Here's the drawing with two shaded views (mm, measured from the low corner). I have some questions. A direction names the side the tool comes from. Coordinates: 2 decimals unless noted, no trailing zeros. Loops run counter-clockwise (first coordinate to the right, second up) from the corner with the lowest first, then second, coordinate; pieces in that order, holes last. Notation, with made-up numbers: (-32, 7.25) -> (7, 7.25) arc R20 ccw to (7, 41.25) -> close; hole circle Ø10 at (5, 87). An arc over 180 degrees is marked (long way). Answer as a JSON object with one key per item and string values. Group by question number.
Q1. I want a section at C-C on y = 22. Write out the boundary of the cut face in (x, z).
Q2. I want a section at A-A on x = 26. Write out the boundary of the cut face in (y, z) (1 decimal), then the cut area to 3 significant figures.
Q3. On a 3-axis mill with a long thin cutter (end or side, diameter ignored), from which of +Z, -Z, +X, -X, +Y, -Y can I reach the whole of each face in a straight line? I mean the marked faces 1 and 2. Say none if no direction works.
Q4. I want a section at B-B on z = 11.5. Write out the boundary of the cut face in (x, y), then the cut area to 3 significant figures.
Q5. I want a section at D-D on x = 67. Write out the boundary of the cut face in (y, z) (1 decimal), then the cut area to 3 significant figures.
Q6. I need wall thicknesses on line 1 (Y direction, x = 29.5, z = 40); line 2 (Z direction, x = 21, y = 10); line 3 (X direction, y = 16, z = 22) (1 decimal). Which ranges of each line are inside material? Lowest first, please.
Q7. I'm going to push flat-ended pins straight in: pin 1 (6 mm diameter, centred on x = 49, y = 42.5, fed in from -Z); pin 2 (1 mm diameter, centred on x = 38.5, z = 49, fed in from -Y). Where does each tip first touch, or does it pass through?
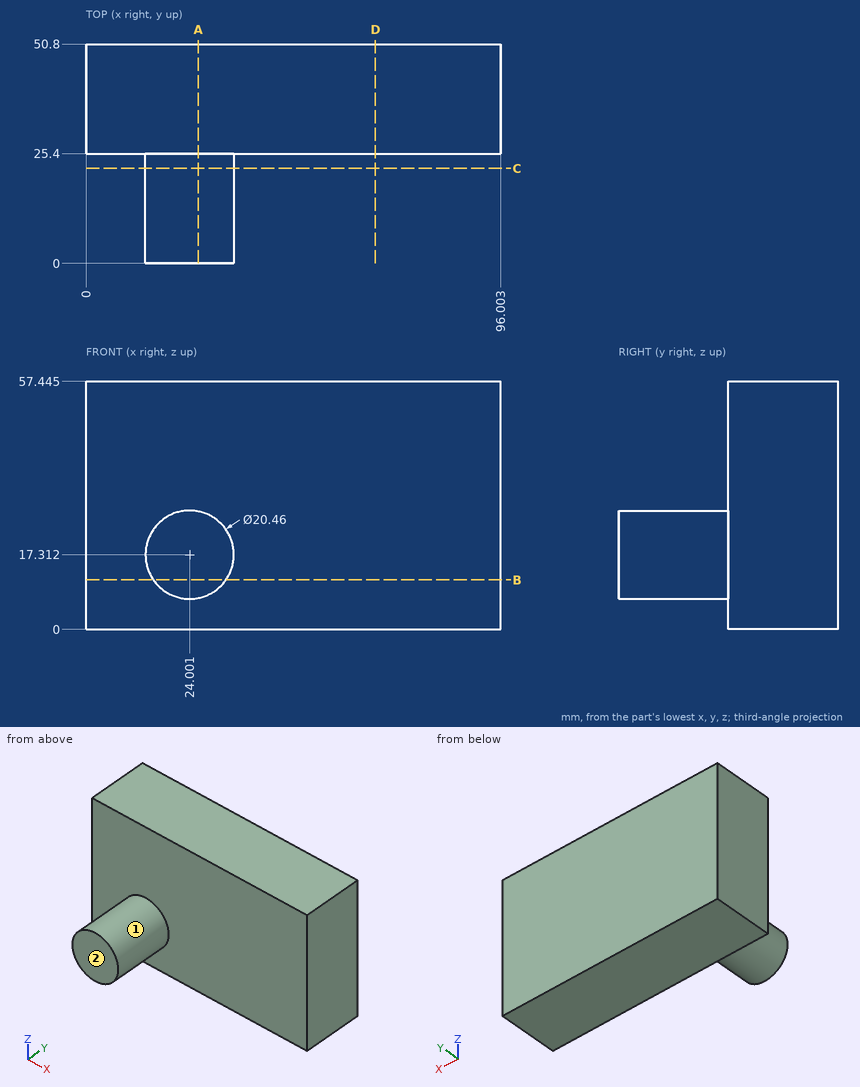
Result set:
{
 "1": {"outline": "circle Ø20.46 at (24, 17.31)"},
 "2": {"outline": "(0, 7.3) -> (25.4, 7.3) -> (25.4, 0) -> (50.8, 0) -> (50.8, 57.4) -> (25.4, 57.4) -> (25.4, 27.3) -> (0, 27.3) -> close", "area": "1,970 mm²"},
 "3": {"face 1": "-Y", "face 2": "+Z, -Z, +X, -X, -Y"},
 "4": {"outline": "(0, 25.4) -> (15.58, 25.4) -> (15.58, 0) -> (32.42, 0) -> (32.42, 25.4) -> (96, 25.4) -> (96, 50.8) -> (0, 50.8) -> close", "area": "2,870 mm²"},
 "5": {"outline": "(25.4, 0) -> (50.8, 0) -> (50.8, 57.4) -> (25.4, 57.4) -> close", "area": "1,460 mm²"},
 "6": {"line 1": "y = 25.4 to 50.8", "line 2": "z = 7.53 to 27.09", "line 3": "x = 14.9 to 33.1"},
 "7": {"pin 1": "stops at z = 0", "pin 2": "stops at y = 25.4"}
}
